Could you check a few things on this model? Use its own coordinates, in mm. A direction names the side the tool comes from. Coordinates: 2 decimals unless noted, no trailing zeros. Loops run counter-clockwise (first coordinate to the right, second up) from the corner with the lowest first, then second, coordinate; pieces in that order, holes last.
1) If I drill on line 1 along Z through (x, y) = (0, 17.5); line 2 along Y through (x, z) = (-2.5, -4.5); line 3 along X through (y, z) = (14, 0.75), over which ranges is the centre line in solid material (lowest first)?
2) Thinking about a two-plate mould opening in Z: for faces 3 (the face through (1, 21.519, -1)), 4 (the face through (2.19, 11.75, 0.69)), 5 (the face through (1.14, 11.39, -0.36)), 6 (the face through (0, 0.973, 0)), which applies, released by +Z, released by -Z, zero draft, split by the parting line, or undercut?
3) For faces 1 (the face through (0, 0, 0)), 2 (the face through (4, 0.973, -1)), which set-ups out of +Z, -Z, +X, -X, +Y, -Y let a thin tool reach every point of the face, with its end or its side?
4) Imagine slicing it at B-B on x = 0. Please give me the cut outline in (y, z), plus the area to 3 significant figures.
5) Will these pins go through, and if not, where does the flat tip stop? P1, Ø6, axis at x = -3.5, z = -3, coming from the +Y side; P2, Ø1, axis at x = 2, y = 9, coming from the -Z side; P3, Ø2, axis at y = 16.5, z = 4.5, coming from the -X side; P4, Ø0.5, axis at x = 4, z = 1.5, coming from the +Y side.
6) Imagine slicing it at A-A on z = 0. Please give me the cut outline in (x, y), plus the area to 3 significant figures.
7) Imagine slicing it at C-C on y = 5.25. Please give me the cut outline in (x, z), plus the area to 3 significant figures.
Autodesk Inventor part; units mm, degrees
ref_plane "YZ Plane" through (0, 0, 0) normal (1, 0, 0) x (0, 1, 0)
ref_plane "XZ Plane" through (0, 0, 0) normal (0, 1, 0) x (-1, 0, 0)
ref_plane "XY Plane" through (0, 0, 0) normal (0, 0, 1) x (1, 0, 0)
sketch "Sketch1" plane through (0, 0, 0) normal (0, 0, 1) x (1, 0, 0)
  line L0 (1.1948, 21.5189) -> (2.2959, 21.5189)
  line L1 (6.6309, 0) -> (1.1948, 0)
  line L2 (1.1948, 0.9728) -> (1.1948, 21.5189)
  line L3 (2.2959, 21.5189) -> (2.2959, 0.9728)
  line L4 (2.2959, 0.9728) -> (6.6309, 0.9728)
  line L5 (6.6309, 0.9728) -> (6.6309, 0)
  line L6 (1.1948, 0.9728) -> (0, 0.9728)
  line L7 (0, 0.9728) -> (0, 0)
  line L8 (0, 0) -> (1.1948, 0)
revolve "Revolution1" add sketch "Sketch1" angle 360 about axis through (0, 0.9728, 0) along (0, -1, 0)
fillet "Fillet1" radius 1.27 1 edges at (-2.2959, 0.9728, 0)
fillet "Fillet2" radius 1.27 1 edges at (-6.6309, 0.9728, 0)
sketch "Sketch2" plane through (0, 0.9728, 0) normal (0, 1, 0) x (1, 0, 0)
  circle A0 centre (0, 0) radius 3.5659
  circle A1 centre (0, 0) radius 5.3961
  circle A2 centre (-0.0164, -4.5633) radius 0.3175
  circle A3 centre (1.841, -4.1755) radius 0.3175
  circle A4 centre (3.3802, -3.0657) radius 0.3175
  circle A5 centre (4.3349, -1.4258) radius 0.3175
  circle A6 centre (4.54, 0.4606) radius 0.3175
  circle A7 centre (3.9602, 2.2674) radius 0.3175
  circle A8 centre (2.6955, 3.6821) radius 0.3175
  circle A9 centre (0.9648, 4.4602) radius 0.3175
  circle A10 centre (-0.9327, 4.467) radius 0.3175
  circle A11 centre (-2.6689, 3.7015) radius 0.3175
  circle A12 centre (-3.9437, 2.2959) radius 0.3175
  circle A13 centre (-4.5366, 0.4933) radius 0.3175
  circle A14 centre (-4.345, -1.3945) radius 0.3175
  circle A15 centre (-3.4022, -3.0412) radius 0.3175
  circle A16 centre (-1.8711, -4.1621) radius 0.3175
  point P0 (0, 0)
  dimension "d3" = 0.635
  dimension "d6" = 360
extrude "Extrusion1" add sketch "Sketch2" along normal blind 1.27 contours A15
pattern_circular "Circular Pattern1" count 6 over 360 about axis through (0, -10, 0) along (0, 1, 0) of "Extrusion1"
properties part number "flume-nursery"
Filled in:
1. line 1: z = -2.3 to -1.19, 1.19 to 2.3
1. line 2: y = 0 to 0.97
1. line 3: x = -2.17 to -0.93, 0.93 to 2.17
2. face 3: zero draft
2. face 4: split by the parting line
2. face 5: undercut
2. face 6: undercut
3. face 1: +Z, -Z, +X, -X, -Y
3. face 2: +Y
4. outline: (0, -6.63) arc R1.27 ccw to (0.97, -5.4) - (0.97, -3.57) arc R1.27 cw to (2.24, -2.3) - (21.52, -2.3) - (21.52, -1.19) - (0.97, -1.19) - (0.97, 1.19) - (21.52, 1.19) - (21.52, 2.3) - (2.24, 2.3) arc R1.27 cw to (0.97, 3.57) - (0.97, 5.4) arc R1.27 ccw to (0, 6.63) - close
4. area: 58.2 mm2
5. P1: stops at y = 21.52
5. P2: stops at z = -1.74
5. P3: passes through
5. P4: stops at y = 2.24
6. outline: (-6.63, 0) - (6.63, 0) arc R1.27 ccw to (5.4, 0.97) - (3.57, 0.97) arc R1.27 cw to (2.3, 2.24) - (2.3, 21.52) - (1.19, 21.52) - (1.19, 0.97) - (-1.19, 0.97) - (-1.19, 21.52) - (-2.3, 21.52) - (-2.3, 2.24) arc R1.27 cw to (-3.57, 0.97) - (-5.4, 0.97) arc R1.27 ccw to start
6. area: 58.2 mm2
7. outline: circle Ø4.59 at (0, 0); hole circle Ø2.39 at (0, 0)
7. area: 12.1 mm2
